```python
from build123d import *

# Parameters (mm, degrees)
F0_R     = 25.3953088791
F1_DEPTH = 111
F2_T     = -9
F3_R     = 3.1384776311


with BuildPart() as f1:
    # F0 (on Top) → F1 (new body)
    with BuildSketch(Plane.XY):
        Circle(F0_R)
    extrude(amount=F1_DEPTH)

    # F2
    f2_openings = [f1.faces().sort_by_distance(p)[0] for p in [
        (0, 0, 111),
    ]]
    offset(amount=F2_T, openings=f2_openings)

    # F3
    f3_edges = [f1.edges().sort_by_distance(p)[0] for p in [
        (25.395309, 0, 55.5),
        (-25.395309, 0, 0),
        (-25.395309, 0, 111),
        (-16.395309, 0, 9),
    ]]
    fillet(f3_edges, radius=F3_R)


solid = f1.part
```
The model under review builds one solid part; all positions refer to its coordinate system, in mm. Round coordinates to 2 decimals unless told otherwise and drop trailing zeros. Write each loop counter-clockwise with the first axis right and the second up, starting at its lowest first coordinate (ties: lowest second). Pieces come first, ordered by that corner, then holes.
(1) We need section C-C on z = 55. Give the boundary of the cut face in (x, y).
(2) Insertion check: pin 1 (1.5 mm diameter, centred on x = -14.5, z = 39, fed in from -Y); pin 2 (8 mm diameter, centred on x = -5, z = 63.5, fed in from +Y); pin 3 (6 mm diameter, centred on x = -8.5, y = -2, fed in from +Z). Each pin has a flat end and moves straight along its axis. Give the tip position at first contact, or say it passes through.
(3) Mouldability with a two-part tool opening along Y and no side actions: class faces 1 (the cylindrical face through (24.22, 7.63, 54.77)), 2 (the flat face through (0, 0, 9)), 3 (the cylindrical face through (-3.554, -16.005, 60.877)), 4 (the flat face through (-8, -15, 111)) as +Y half, -Y half, draft (parallel to the pull), parting line (faces both ways), or undercut.
(4) We need section A-A on x = 0. Give the boundary of the cut face in (y, z), and give its area (3 significant figures).
(5) Wall thickness on L1, parallel to Y at x = 0, z = 49; L2, parallel to Z at x = 0.5, y = 5; L3, parallel to Y at x = -11, z = 90.5: over which ranges is each line inside the solid? List them lowest first.
(6) We need section D-D on z = 11. Give the boundary of the cut face in (x, y).
Findings below:
1. outline: circle Ø50.79 at (0, 0); hole circle Ø32.79 at (0, 0)
2. pin 1: stops at y = -21.35
2. pin 2: stops at y = 25.38
2. pin 3: stops at z = 9
3. face 1: parting line
3. face 2: undercut
3. face 3: undercut
3. face 4: draft
4. outline: (-25.4, 3.14) arc R3.14 ccw to (-22.26, 0) - (22.26, 0) arc R3.14 ccw to (25.4, 3.14) - (25.4, 107.86) arc R3.14 ccw to (22.26, 111) - (16.4, 111) - (16.4, 12.14) arc R3.14 cw to (13.26, 9) - (-13.26, 9) arc R3.14 cw to (-16.4, 12.14) - (-16.4, 111) - (-22.26, 111) arc R3.14 ccw to (-25.4, 107.86) - close
4. area: 2,290 mm2
5. L1: y = -25.4 to -16.4, 16.4 to 25.4
5. L2: z = 0 to 9
5. L3: y = -22.89 to -12.16, 12.16 to 22.89
6. outline: circle Ø50.79 at (0, 0); hole circle Ø32.36 at (0, 0)
